Study the drawing (mm; zero at the part's minimum x, y, z) and answer. Give positions to 0.01 mm unless a question says otherwise; leave off trailing zeros. Loops run counter-clockwise (first coordinate to the right, second up) from the corner with the lowest first, then second, coordinate; pieces in that order, holes last. Notation, with made-up numbers: M -13.5,11 L -7.5,11 A33 ccw -7.5,48 Z; hole C -8.5,3.5 d2. An arc over 180 degrees is marked long. Use one line per item in the form item = value. Start each with the question number.
1. Each of these flat-tipped pins is pushed along its axis until it touches: pin 1 Ø0.9 at (x, y) = (27, 2) entering from -Z; pin 2 Ø1.5 at (y, z) = (1, 56) entering from +X; pin 3 Ø1.5 at (x, y) = (25.5, 1) entering from +Z. Where does it stop, or does it pass through?
2. The part is cut by section A-A (x = 8.5). Write down the section's boundary in (y, z).
3. Straight lines are drawn through the part: line 1 (X direction, y = 0.95, z = 55); line 2 (Y direction, x = 18, z = 1.5); line 3 (Z direction, x = 28, y = 1.45). For each, find the intervals that lie inside material, in ascending order. Write a range as from..to.
4. The part is cut by section B-B (x = 26). Write down the section's boundary in (y, z).
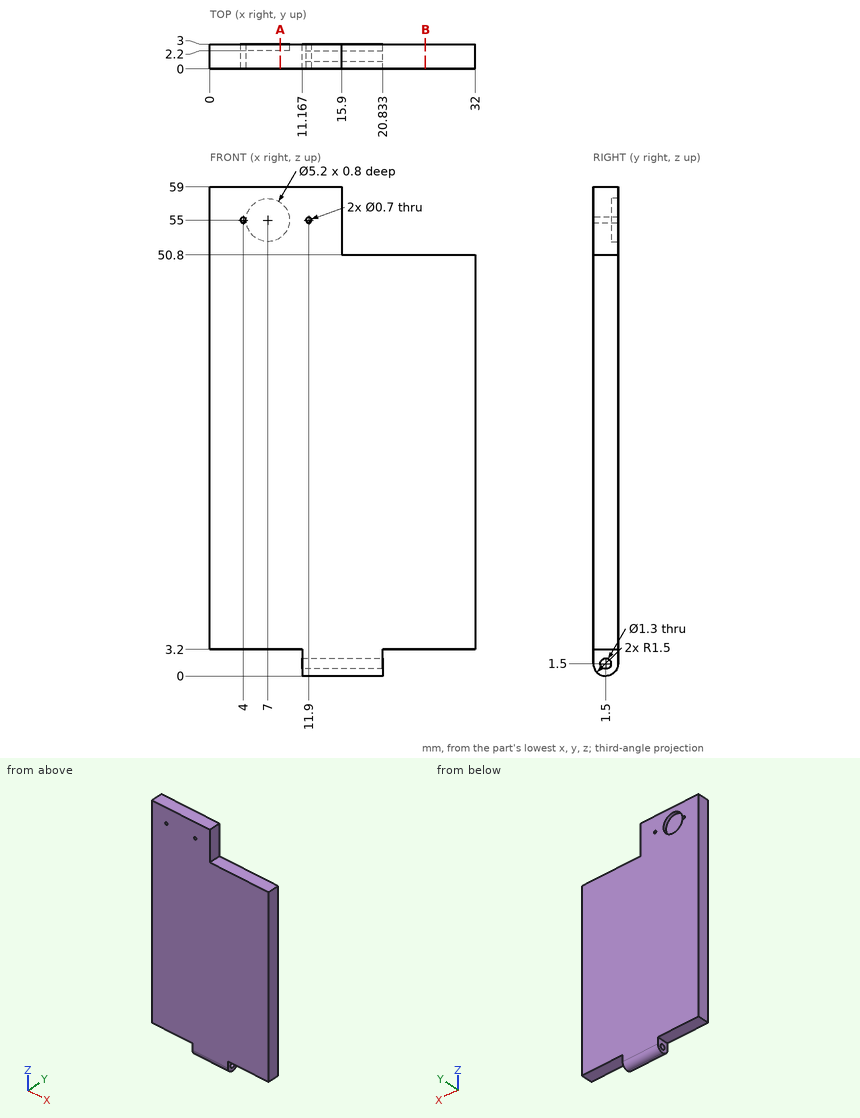
Derived:
q1.pin_1 = 3.2
q1.pin_2 = 15.9
q1.pin_3 = 50.8
q2.outline = M 0,3.2 L 3,3.2 L 3,52.88 L 2.2,52.88 L 2.2,57.12 L 3,57.12 L 3,59 L 0,59 Z
q3.line_1 = 0..3.65, 4.35..11.55, 12.25..15.9
q3.line_2 = 0..0.85, 2.15..3
q3.line_3 = 3.2..50.8
q4.outline = M 0,3.2 L 3,3.2 L 3,50.8 L 0,50.8 Z
